The listing builds one solid part. Answer for the finished solid, in the listing's coordinates (mm). A direction names the side the tool comes from. Round coordinates to 2 decimals unless told otherwise and drop trailing zeros. Order: outer loops, then holes, each group sorted by start corner. A loop starts at its lowest first (then second) coordinate and runs counter-clockwise, first axis right, second up. Notation, with made-up numbers: (67.5, -11.75) - (111.5, -11.75) arc R17 cw to (111.5, 1.25) - close; hole circle Ø5 at (2.25, -5.75). An arc over 180 degrees is marked (long way). Use CSV: the item, a comma, the result in double quotes. Start each with the question number.
Item 1: For faces 4 (the flat face through (-6, -89.273, -17)), 5 (the flat face through (0, -97.273, 0)), determine the directions among +Z, -Z, +X, -X, +Y, -Y from which every point of the face is accessible in a straight line to the end or side of a thin tool.
Item 2: Straight lines are drawn through the part: line 1 along X through (y, z) = (-58, 0); line 2 along Y through (x, z) = (17, 10.5); line 3 along X through (y, z) = (-73.5, 2). For each, find the intervals that lie inside material, in ascending order. Write a range as [from, to].
Item 3: Flat-ended cylindrical pins translate along their axes: P1, Ø1.5, axis at y = -79, z = -10, coming from the -X side; P2, Ø1, axis at x = 0, y = -70, coming from the -Z side; P3, Ø5, axis at y = -68, z = 14, coming from the +X side. Find the tip coordinate at first contact, or state that the pin passes through.
Item 4: Find section C-C, the plane y = -82.5. Give the vertices of the cut face in (x, z), plus the area to 3 significant figures.
Item 5: Find section D-D, the plane x = 15.5. Give the vertices of the cut face in (y, z).
Item 6: Find section B-B, the plane y = -67.5. Give the vertices of the cut face in (x, z), plus the area to 3 significant figures.
Item 7: Find section A-A, the plane z = -7.5. Give the vertices of the cut face in (x, y).
Item 8: Determine the mould class of faces 1 (the flat face through (8, -43.793, 0)), 2 (the cylindrical face through (-7.36, -93.22, 23.37)), 3 (the cylindrical face through (5.96, -58.58, -1.88)) for opening direction X: +X half, -X half, draft (parallel to the pull), parting line (faces both ways), or undercut.
```python
from build123d import *


# Read off the part's stored shape, not the designer's step: PerçageAvancé1
with BuildPart() as part:
    # Esquisse1 → Révolution1 (revolve)
    with BuildSketch(Plane.XY, mode=Mode.PRIVATE) as r_volution1_sk:
        Polygon((0, -43.792727273), (0, -97.272727273), (-24.5, -97.272727273), (-24.5, -89.272727273), (-17.5, -89.272727273), (-17.5, -43.792727273), align=None)
    revolve(r_volution1_sk.sketch.rotate(Axis((0, 115.909090909, 0), (0, -1, 0)), 270), axis=Axis((0, 115.909090909, 0), (0, -1, 0)))

    # PerçageAvancé1 outline → PerçageAvancé1 (revolve, cut)
    with BuildSketch(Plane.XY):
        Polygon((0, -77.548106142), (6.25, -73.792727273), (6.25, -43.792727273), (0, -43.792727273), align=None)
    revolve(axis=Axis((0, 0, 0), (0, 1, 0)), mode=Mode.SUBTRACT)


solid = part.part
```
Worked out:
1,face 4,"+Y"
1,face 5,"+Z, -Z, +X, -X, -Y"
2,line 1,"x = [-17.5, -6.25], [6.25, 17.5]"
2,line 2,"y = [-97.27, -89.27]"
2,line 3,"x = [-17.39, -5.92], [5.92, 17.39]"
3,P1,"stops at x = -14.86"
3,P2,"stops at z = -17.5"
3,P3,"stops at x = 13.19"
4,outline,"circle Ø35 at (0, 0)"
4,area,"962 mm²"
5,outline,"(-97.27, -18.97) - (-89.27, -18.97) - (-89.27, -8.12) - (-43.79, -8.12) - (-43.79, 8.12) - (-89.27, 8.12) - (-89.27, 18.97) - (-97.27, 18.97) - close"
6,outline,"circle Ø35 at (0, 0); hole circle Ø12.5 at (0, 0)"
6,area,"839 mm²"
7,outline,"(-23.32, -97.27) - (23.32, -97.27) - (23.32, -89.27) - (15.81, -89.27) - (15.81, -43.79) - (-15.81, -43.79) - (-15.81, -89.27) - (-23.32, -89.27) - close"
8,face 1,"draft"
8,face 2,"parting line"
8,face 3,"undercut"
